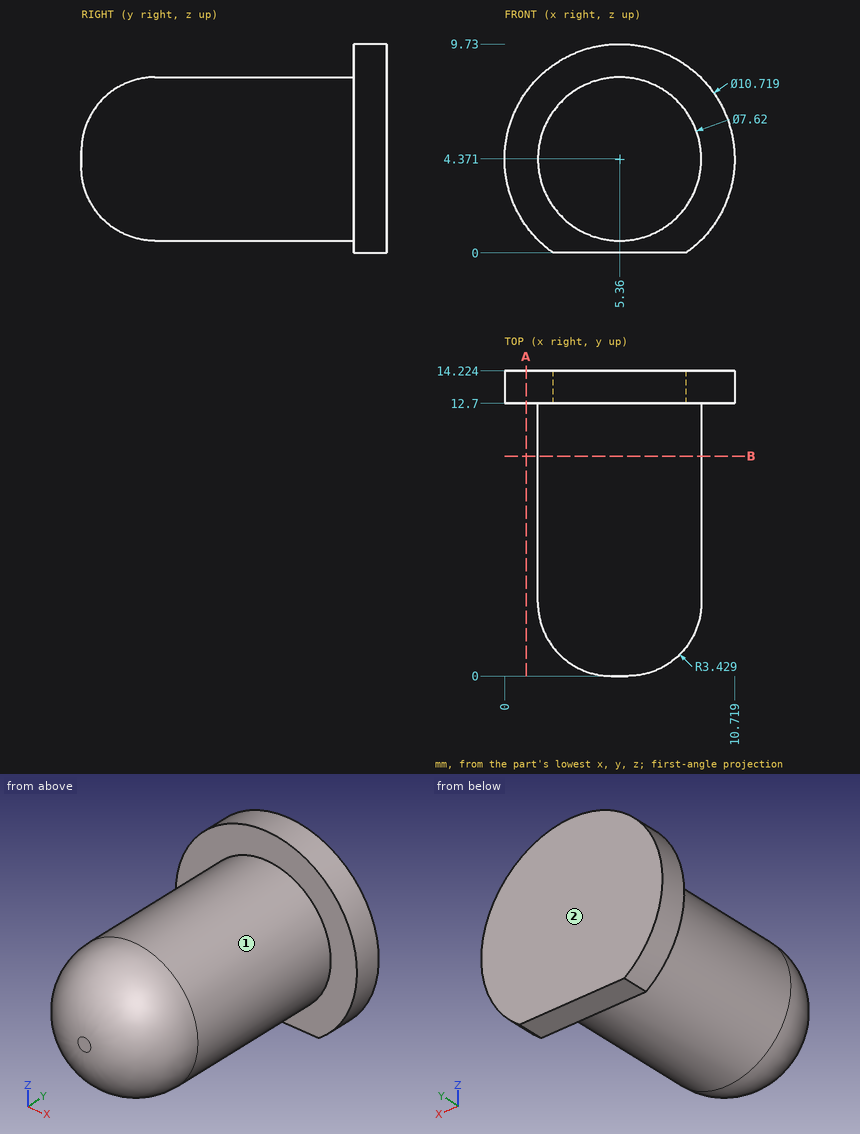
Can you work these out from the drawing? Everything is in mm from the part's minimum corner. A direction names the side the tool comes from. Give positions to 0.01 mm unless a question says otherwise; leave off trailing zeros. Loops run counter-clockwise (first coordinate to the right, second up) from the corner with the lowest first, then second, coordinate; pieces in that order, holes last. Notation, with made-up numbers: (63, 83.5) -> (80, 83.5) arc R21 cw to (80, 93.5) -> close; hole circle Ø9 at (83, 71.25). An arc over 180 degrees is marked (long way). Return JSON: item names as keys, results as strings.
Item 1: I'm going to push flat-ended pins straight in: pin 1 (4 mm diameter, centred on x = 3.5, y = 10, fed in from -Z); pin 2 (1.5 mm diameter, centred on y = 11.5, z = 3.5, fed in from +X); pin 3 (1.5 mm diameter, centred on x = 2, z = 5, fed in from -Y) (1 decimal). Where does each tip first touch, or does it pass through?
Geometry results:
{"pin 1": "stops at z = 0.56", "pin 2": "stops at x = 9.17", "pin 3": "stops at y = 0.9"}
Item 2: If we section it at A-A on x = 1: List the corners of the cut face in (y, z) for me.
Geometry results:
{"outline": "(12.7, 1.25) -> (14.22, 1.25) -> (14.22, 7.49) -> (12.7, 7.49) -> close"}
Item 3: If we section it at B-B on y = 10.25: List the corners of the cut face in (x, z) for me, plus the area to 3 significant figures.
Geometry results:
{"outline": "circle Ø7.62 at (5.36, 4.37)", "area": "45.6 mm²"}
Item 4: I need wall thicknesses on L1, parallel to Y at x = 8, z = 8.25; L2, parallel to X at y = 4.25, z = 4.5; L3, parallel to Y at x = 5, z = 5.75 (1 decimal). Which ranges of each line are inside material? Lowest first, please. Write a range as from..to.
Geometry results:
{"L1": "y = 12.7..14.22", "L2": "x = 1.55..9.17", "L3": "y = 0.2..14.2"}
Item 5: Which directions (+Z, -Z, +X, -X, +Y, -Y) give clear straight access to the entire face, cutting with the end or side of a thin tool? Please do the marked faces 1 and 2.
Geometry results:
{"face 1": "-Y", "face 2": "+Z, -Z, +X, -X, +Y"}
